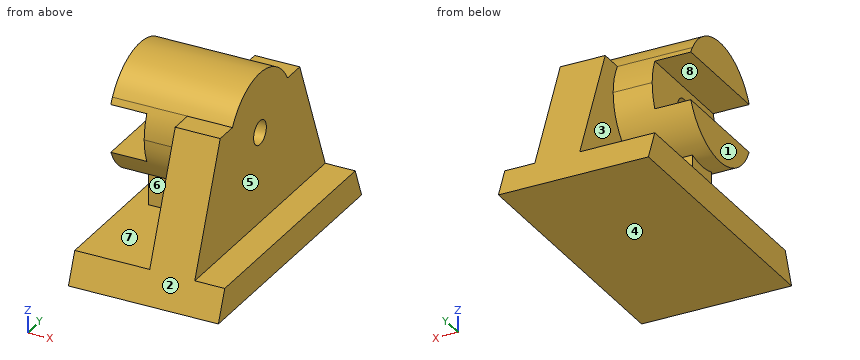
from build123d import *

# Parameters (mm, degrees)
F0_W          = 50
F0_H          = 10
F1_DEPTH      = 25
F2_DEPTH      = 15
F3_DEPTH      = 15
F3_DEPTH_BACK = 25
F5_DEPTH      = 12
F6_D          = 8
F7_W          = 19
F7_H          = 12
F8_DEPTH      = 25


with BuildPart() as f1:
    # F0 (on Right) → F1 (new body, symmetric)
    with BuildSketch(Plane.YZ):
        Polygon((41, -15), (25, -15), (25, -25), (45, -25), align=None)
        with Locations((0, -20)):
            Rectangle(F0_W, F0_H)
        Polygon((-25, -15), (-41, -15), (-45, -25), (-25, -25), align=None)
    extrude(amount=F1_DEPTH, both=True)

    # F0 (on Right) → F2 (join)
    with BuildSketch(Plane.YZ):
        with BuildLine():
            Line((-20, 15), (-25, 15))
            Line((-25, 15), (-25, -15))
            Line((-25, -15), (25, -15))
            Line((25, -15), (25, 15))
            Line((25, 15), (20, 15))
            ThreePointArc((20, 15), (0, -5), (-20, 15))
        make_face()
        Polygon((41, -15), (25, 25), (25, 15), (25, -15), align=None)
        Polygon((-25, 15), (-25, 25), (-41, -15), (-25, -15), align=None)
        with BuildLine():
            Line((-17.3205080757, 25), (-25, 25))
            Line((-25, 25), (-25, 15))
            Line((-25, 15), (-20, 15))
            ThreePointArc((-20, 15), (-19.3185165258, 20.1763809021), (-17.3205080757, 25))
        make_face()
        with BuildLine():
            Line((25, 25), (17.3205080757, 25))
            ThreePointArc((17.3205080757, 25), (19.3185165258, 20.1763809021), (20, 15))
            Line((20, 15), (25, 15))
            Line((25, 15), (25, 25))
        make_face()
    extrude(amount=F2_DEPTH)

    # F0 (on Right) → F3 (join, two sides)
    with BuildSketch(Plane.YZ) as f3_sk:
        with BuildLine():
            ThreePointArc((17.3205080757, 25), (0, 35), (-17.3205080757, 25))
            Line((-17.3205080757, 25), (17.3205080757, 25))
        make_face()
        with BuildLine():
            Line((17.3205080757, 25), (-17.3205080757, 25))
            ThreePointArc((-17.3205080757, 25), (-19.3185165258, 20.1763809021), (-20, 15))
            Line((-20, 15), (20, 15))
            ThreePointArc((20, 15), (19.3185165258, 20.1763809021), (17.3205080757, 25))
        make_face()
        with BuildLine():
            Line((20, 15), (-20, 15))
            ThreePointArc((-20, 15), (0, -5), (20, 15))
        make_face()
    extrude(amount=F3_DEPTH)
    extrude(f3_sk.sketch, amount=-F3_DEPTH_BACK)

    # F4 (on face) → F5 (cut)
    with BuildSketch(Plane(origin=(-25, 0, 0), x_dir=(0, -1, 0), z_dir=(-1, 0, 0))):
        with BuildLine():
            ThreePointArc((20, 15), (19.5781262586, 19.0861928738), (18.3303027798, 23))
            Line((18.3303027798, 23), (-18.3303027798, 23))
            ThreePointArc((-18.3303027798, 23), (-19.5781262586, 19.0861928738), (-20, 15))
            Line((-20, 15), (20, 15))
        make_face()
        with BuildLine():
            ThreePointArc((18.3303027798, 7), (19.5781262586, 10.9138071262), (20, 15))
            Line((20, 15), (-20, 15))
            ThreePointArc((-20, 15), (-19.5781262586, 10.9138071262), (-18.3303027798, 7))
            Line((-18.3303027798, 7), (18.3303027798, 7))
        make_face()
    extrude(amount=-F5_DEPTH, mode=Mode.SUBTRACT)

    # F6 (through all)
    with Locations(Plane(origin=(-25, 0, 0), x_dir=(0, -1, 0), z_dir=(-1, 0, 0))):
        with Locations((0, 15)):
            Hole(F6_D / 2)

    # F7 (on Top) → F8 (join)
    with BuildSketch(Plane.XY):
        with Locations((-9.5, 0)):
            Rectangle(F7_W, F7_H)
    extrude(amount=-F8_DEPTH)


solid = f1.part
Source: CAD feature listing. Evaluate the final solid. Frame: model axes, mm. Face numbers are marked on the shaded views. A direction names the side the tool comes from. Round coordinates to 2 decimals unless told otherwise and drop trailing zeros. Write each loop counter-clockwise with the first axis right and the second up, starting at its lowest first coordinate (ties: lowest second). Pieces come first, ordered by that corner, then holes. Notation, with made-up numbers: M 63.25,83.5 L 87.25,83.5 A19 ccw 87.25,100.5 Z; hole C -35,53.25 d2. An arc over 180 degrees is marked long. One line per item, written item: value. Start each with the question number.
Item 1: Ray query, L1, parallel to Z at x = 1.75, y = 0; L2, parallel to Z at x = -20.5, y = -4; L3, parallel to Z at x = -14, y = -13.5. Return the intervals inside material, ascending. Write a range as from..to.
Item 2: Section query D-D (y = 36). Return the cut outline in (x, z).
Item 3: Set-up query: the marked faces 4, 5, 6, 7 and 8. Return all of +Z, -Z, +X, -X, +Y, -Y with unobstructed straight access to the full face (end or side cutting, diameter ignored); none if empty.
Item 4: Pin query (flat end, axial travel): pin 1 (15 mm diameter, centred on y = -17.5, z = 15.5, fed in from +X); pin 2 (8.5 mm diameter, centred on x = -14, z = -8.5, fed in from +Y); pin 3 (5.5 mm diameter, centred on y = 2.5, z = -12, fed in from -X). Return the tip coordinate at first contact, or that it passes through.
Item 5: Section query A-A (x = 14). Return the cut outline in (y, z), plus the area to 3 significant figures.
Item 6: Section query B-B (y = 0). Return the cut outline in (x, z).
Item 7: Mould query, pull axis Z, two halves, no side actions, for the marked faces 1, 2 and 3. Classes: pulls with the +Z half, pulls with the -Z half, needs draft (parallel to the pull), parting line crosses it, or undercut.
Item 8: Section query C-C (z = -13). Return the cut outline in (x, y).
Result set:
1. L1: z = -25..11, 19..35
1. L2: z = -25..-15, -4.6..7, 23..34.6
1. L3: z = -25..-15, 0.24..7, 23..29.76
2. outline: M -25,-25 L 25,-25 L 25,-15 L 15,-15 L 15,-2.5 L 0,-2.5 L 0,-15 L -25,-15 Z
3. face 4: -Z, +X, -X, +Y, -Y
3. face 5: +Z, +X, +Y, -Y
3. face 6: -X, -Y
3. face 7: -X
3. face 8: -X, +Y, -Y
4. pin 1: stops at x = 15
4. pin 2: stops at y = 6
4. pin 3: stops at x = -19
5. outline: M -45,-25 L 45,-25 L 25,25 L 17.32,25 A20 ccw -17.32,25 L -25,25 Z; hole C 0,15 d8
5. area: 3,700 mm²
6. outline: M -25,-25 L 25,-25 L 25,-15 L 15,-15 L 15,11 L -13,11 L -13,7 L -25,7 L -25,-5 L -19,-5 L -19,-15 L -25,-15 Z; M -25,23 L -13,23 L -13,19 L 15,19 L 15,35 L -25,35 Z
7. face 1: needs draft
7. face 2: pulls with the +Z half
7. face 3: undercut
8. outline: M -19,-6 L 0,-6 L 0,-40.2 L 15,-40.2 L 15,40.2 L 0,40.2 L 0,6 L -19,6 Z
